```python
from build123d import *

# Parameters (mm, degrees)
SKETCH1_R             = 92.5
BOSS_EXTRUDE1_DEPTH   = 6
SKETCH2_R             = 10
CUT_EXTRUDE1_DEPTH    = 131.952281385
SKETCH3_R             = 10
CUT_EXTRUDE2_DEPTH    = 4.941973
CIRPATTERN1_START     = 1.058026988
CIRPATTERN1_OUTLINE_R = 10
CIRPATTERN1_DEPTH     = 4.941973012


# Read off the part's stored shape, not the designer's step: CirPattern1
with BuildPart() as part:
    # Sketch1 → Boss-Extrude1 (new body)
    with BuildSketch(Plane(origin=(0, 0, 0), x_dir=(1, 0, 0), z_dir=(0, 1, 0))):
        with Locations(Location((0, 0, 0), (0, 0, 270))):
            Circle(SKETCH1_R)
    extrude(amount=BOSS_EXTRUDE1_DEPTH)

    # Sketch2 → Cut-Extrude1 (cut, through all)
    with BuildSketch(Plane(origin=(0, 0, 0), x_dir=(1, 0, 0), z_dir=(0, 1, 0))):
        with Locations(Location((0, 0, 0), (0, 0, 270))):
            Circle(SKETCH2_R)
    extrude(amount=CUT_EXTRUDE1_DEPTH, mode=Mode.SUBTRACT)

    # Sketch3 → Cut-Extrude2 (cut)
    with BuildSketch(Plane(origin=(0, 6, 0), x_dir=(1, 0, 0), z_dir=(0, 1, 0))):
        with Locations(Location((-30.914776162, 0, 0), (0, 0, 270))):
            Circle(SKETCH3_R)
    extrude(amount=-CUT_EXTRUDE2_DEPTH, mode=Mode.SUBTRACT)

    # CirPattern1 outline → CirPattern1 (cut)
    with BuildSketch(Plane(origin=(0, 0, 0), x_dir=(1, 0, 0), z_dir=(0, 1, 0)).offset(CIRPATTERN1_START)):
        with Locations((-9.553191211, -29.401699319)):
            Circle(CIRPATTERN1_OUTLINE_R)
        with Locations((25.010579293, -18.171249506)):
            Circle(CIRPATTERN1_OUTLINE_R)
        with Locations((25.010579293, 18.171249506)):
            Circle(CIRPATTERN1_OUTLINE_R)
        with Locations((-9.553191211, 29.401699319)):
            Circle(CIRPATTERN1_OUTLINE_R)
    extrude(amount=CIRPATTERN1_DEPTH, mode=Mode.SUBTRACT)


solid = part.part
```
Here's how the part is built. I have some questions about the finished solid (model axes, mm). A direction names the side the tool comes from. Coordinates: 2 decimals unless noted, no trailing zeros. Loops run counter-clockwise (first coordinate to the right, second up) from the corner with the lowest first, then second, coordinate; pieces in that order, holes last. Notation, with made-up numbers: (-27.5, 23) -> (12.5, 23) arc R29 ccw to (12.5, 61) -> close; hole circle Ø1 at (17, -32.75). An arc over 180 degrees is marked (long way). Return JSON: item names as keys, results as strings.
1) If we section it at B-B, the plane x = -6: Write out the boundary of the cut face in (y, z), then the cut area to 3 significant figures.
Results below:
{"outline": "(0, -92.31) -> (6, -92.31) -> (6, -38.75) -> (1.06, -38.75) -> (1.06, -20.05) -> (6, -20.05) -> (6, -8) -> (0, -8) -> close; (0, 8) -> (6, 8) -> (6, 20.05) -> (1.06, 20.05) -> (1.06, 38.75) -> (6, 38.75) -> (6, 92.31) -> (0, 92.31) -> close", "area": "827 mm²"}
2) If we section it at D-D, the plane z = 22: Write out the boundary of the cut face in (x, y).
Results below:
{"outline": "(-89.85, 0) -> (89.85, 0) -> (89.85, 6) -> (34.25, 6) -> (34.25, 1.06) -> (15.77, 1.06) -> (15.77, 6) -> (-2.83, 6) -> (-2.83, 1.06) -> (-16.28, 1.06) -> (-16.28, 6) -> (-89.85, 6) -> close"}
3) I need wall thicknesses on line 1 (X direction, y = 3.95, z = 0); line 2 (Z direction, x = 1, y = 4.6); line 3 (X direction, y = 1.9, z = -24). Which ranges of each line are inside material? Lowest first, please. Write a range as from..to.
Results below:
{"line 1": "-92.5..-40.91, -20.91..-10, 10..92.5", "line 2": "-92.49..-9.95, 9.95..92.49", "line 3": "-89.33..-17.97, -1.14..16.88, 33.14..89.33"}
4) Thinking about a two-plate mould opening in X: for faces 1 (the face through (-19, 0, -1)), 2 (the face through (25, 1.058, -18)), 3 (the face through (-90.3, 2.96, -20.05)), 4 (the face through (-4.177, 3.494, -37.834)), which applies, +X half, -X half, draft (parallel to the pull), parting line (faces both ways), or undercut?
Results below:
{"face 1": "draft", "face 2": "undercut", "face 3": "parting line", "face 4": "undercut"}
5) For faces 5 (the face through (-11.721, 3.494, 39.164)), 6 (the face through (-19, 6, -1)), which set-ups out of +Z, -Z, +X, -X, +Y, -Y let a thin tool reach every point of the face, with its end or its side?
Results below:
{"face 5": "+Y", "face 6": "+Z, -Z, +X, -X, +Y"}
6) Will these pins go through, and if not, where does the flat tip stop? pin 1 (5 mm diameter, centred on x = -15, z = 46.5, fed in from -Y); pin 2 (6 mm diameter, centred on x = -11, z = 25, fed in from +Y); pin 3 (2 mm diameter, centred on y = 2, z = -45.5, fed in from -X); pin 4 (1.5 mm diameter, centred on y = 2, z = -28.5, fed in from -X).
Results below:
{"pin 1": "y = 0", "pin 2": "y = 1.06", "pin 3": "x = -81.09", "pin 4": "x = -88.24"}
7) If we section it at C-C, the plane y = 2: Write out the boundary of the cut face in (x, z), then the cut area to 3 significant figures.
Results below:
{"outline": "circle Ø185 at (0, 0); hole circle Ø20 at (-30.91, 0); hole circle Ø20 at (-9.55, -29.4); hole circle Ø20 at (-9.55, 29.4); hole circle Ø20 at (0, 0); hole circle Ø20 at (25.01, -18.17); hole circle Ø20 at (25.01, 18.17)", "area": "25,000 mm²"}
8) If we section it at A-A, the plane z = 0: Write out the boundary of the cut face in (x, y), then the cut area to 3 significant figures.
Results below:
{"outline": "(-92.5, 0) -> (-10, 0) -> (-10, 6) -> (-20.91, 6) -> (-20.91, 1.06) -> (-40.91, 1.06) -> (-40.91, 6) -> (-92.5, 6) -> close; (10, 0) -> (92.5, 0) -> (92.5, 6) -> (10, 6) -> close", "area": "891 mm²"}
